```python
from build123d import *

# Parameters (mm, degrees)
BOSS_EXTRUDE1_DEPTH = 4
BOSS_EXTRUDE3_DEPTH = 12


with BuildPart() as part:
    # Sketch1 → Boss-Extrude1 (new body)
    with BuildSketch(Plane(origin=(0, 0, 0), x_dir=(1, 0, 0), z_dir=(0, 1, 0))):
        Polygon((75, 12), (90, 12), (90, 0), (0, 0), (0, 12), (60, 12), (60, 17), (75, 17), align=None)
    extrude(amount=BOSS_EXTRUDE1_DEPTH)

    # Sketch2 → Boss-Extrude3 (add)
    with BuildSketch(Plane.XY):
        with BuildLine():
            Line((1.10505422, 5), (1.175606581, 6.27259339))
            ThreePointArc((1.175606581, 6.27259339), (1.382253241, 6.881354819), (1.916787536, 7.238519216))
            ThreePointArc((1.916787536, 7.238519216), (2.451321831, 6.881354819), (2.657968491, 6.27259339))
            Line((2.657968491, 6.27259339), (2.728520852, 5))
            ThreePointArc((2.728520852, 5), (3.728520852, 4), (4.728520852, 5))
            Line((4.728520852, 5), (4.799073212, 6.27259339))
            ThreePointArc((4.799073212, 6.27259339), (5.005719872, 6.881354819), (5.540254167, 7.238519216))
            ThreePointArc((5.540254167, 7.238519216), (6.074788462, 6.881354819), (6.281435122, 6.27259339))
            Line((6.281435122, 6.27259339), (6.351987483, 5))
            ThreePointArc((6.351987483, 5), (7.351987483, 4), (8.351987483, 5))
            Line((8.351987483, 5), (8.422539844, 6.27259339))
            ThreePointArc((8.422539844, 6.27259339), (8.629186504, 6.881354819), (9.163720799, 7.238519216))
            ThreePointArc((9.163720799, 7.238519216), (9.698255094, 6.881354819), (9.904901754, 6.27259339))
            Line((9.904901754, 6.27259339), (9.975454114, 5))
            ThreePointArc((9.975454114, 5), (10.975454114, 4), (11.975454114, 5))
            Line((11.975454114, 5), (12.046006475, 6.27259339))
            ThreePointArc((12.046006475, 6.27259339), (12.252653135, 6.881354819), (12.78718743, 7.238519216))
            ThreePointArc((12.78718743, 7.238519216), (13.321721725, 6.881354819), (13.528368385, 6.27259339))
            Line((13.528368385, 6.27259339), (13.598920746, 5))
            ThreePointArc((13.598920746, 5), (14.598920746, 4), (15.598920746, 5))
            Line((15.598920746, 5), (15.669473107, 6.27259339))
            ThreePointArc((15.669473107, 6.27259339), (15.876119766, 6.881354819), (16.410654062, 7.238519216))
            ThreePointArc((16.410654062, 7.238519216), (16.945188357, 6.881354819), (17.151835017, 6.27259339))
            Line((17.151835017, 6.27259339), (17.222387377, 5))
            ThreePointArc((17.222387377, 5), (18.222387377, 4), (19.222387377, 5))
            Line((19.222387377, 5), (19.292939738, 6.27259339))
            ThreePointArc((19.292939738, 6.27259339), (19.499586398, 6.881354819), (20.034120693, 7.238519216))
            ThreePointArc((20.034120693, 7.238519216), (20.568654988, 6.881354819), (20.775301648, 6.27259339))
            Line((20.775301648, 6.27259339), (20.845854009, 5))
            ThreePointArc((20.845854009, 5), (21.845854009, 4), (22.845854009, 5))
            Line((22.845854009, 5), (22.91640637, 6.27259339))
            ThreePointArc((22.91640637, 6.27259339), (23.123053029, 6.881354819), (23.657587324, 7.238519216))
            ThreePointArc((23.657587324, 7.238519216), (24.19212162, 6.881354819), (24.398768279, 6.27259339))
            Line((24.398768279, 6.27259339), (24.46932064, 5))
            ThreePointArc((24.46932064, 5), (25.46932064, 4), (26.46932064, 5))
            Line((26.46932064, 5), (26.539873001, 6.27259339))
            ThreePointArc((26.539873001, 6.27259339), (26.746519661, 6.881354819), (27.281053956, 7.238519216))
            ThreePointArc((27.281053956, 7.238519216), (27.815588251, 6.881354819), (28.022234911, 6.27259339))
            Line((28.022234911, 6.27259339), (28.092787272, 5))
            ThreePointArc((28.092787272, 5), (29.092787272, 4), (30.092787272, 5))
            Line((30.092787272, 5), (30.163339632, 6.27259339))
            ThreePointArc((30.163339632, 6.27259339), (30.369986292, 6.881354819), (30.904520587, 7.238519216))
            ThreePointArc((30.904520587, 7.238519216), (31.439054883, 6.881354819), (31.645701542, 6.27259339))
            Line((31.645701542, 6.27259339), (31.716253903, 5))
            ThreePointArc((31.716253903, 5), (32.716253903, 4), (33.716253903, 5))
            Line((33.716253903, 5), (33.786806264, 6.27259339))
            ThreePointArc((33.786806264, 6.27259339), (33.993452924, 6.881354819), (34.527987219, 7.238519216))
            ThreePointArc((34.527987219, 7.238519216), (35.062521514, 6.881354819), (35.269168174, 6.27259339))
            Line((35.269168174, 6.27259339), (35.339720535, 5))
            ThreePointArc((35.339720535, 5), (36.339720535, 4), (37.339720535, 5))
            Line((37.339720535, 5), (37.410272895, 6.27259339))
            ThreePointArc((37.410272895, 6.27259339), (37.616919555, 6.881354819), (38.15145385, 7.238519216))
            ThreePointArc((38.15145385, 7.238519216), (38.685988145, 6.881354819), (38.892634805, 6.27259339))
            Line((38.892634805, 6.27259339), (38.963187166, 5))
            ThreePointArc((38.963187166, 5), (39.963187166, 4), (40.963187166, 5))
            Line((40.963187166, 5), (41.033739527, 6.27259339))
            ThreePointArc((41.033739527, 6.27259339), (41.240386186, 6.881354819), (41.774920482, 7.238519216))
            ThreePointArc((41.774920482, 7.238519216), (42.309454777, 6.881354819), (42.516101437, 6.27259339))
            Line((42.516101437, 6.27259339), (42.586653797, 5))
            ThreePointArc((42.586653797, 5), (43.586653797, 4), (44.586653797, 5))
            Line((44.586653797, 5), (44.657206158, 6.27259339))
            ThreePointArc((44.657206158, 6.27259339), (44.863852818, 6.881354819), (45.398387113, 7.238519216))
            ThreePointArc((45.398387113, 7.238519216), (45.932921408, 6.881354819), (46.139568068, 6.27259339))
            Line((46.139568068, 6.27259339), (46.210120429, 5))
            ThreePointArc((46.210120429, 5), (47.210120429, 4), (48.210120429, 5))
            Line((48.210120429, 5), (48.28067279, 6.27259339))
            ThreePointArc((48.28067279, 6.27259339), (48.487319449, 6.881354819), (49.021853745, 7.238519216))
            ThreePointArc((49.021853745, 7.238519216), (49.55638804, 6.881354819), (49.763034699, 6.27259339))
            Line((49.763034699, 6.27259339), (49.83358706, 5))
            ThreePointArc((49.83358706, 5), (50.83358706, 4), (51.83358706, 5))
            Line((51.83358706, 5), (51.904139421, 6.27259339))
            ThreePointArc((51.904139421, 6.27259339), (52.110786081, 6.881354819), (52.645320376, 7.238519216))
            ThreePointArc((52.645320376, 7.238519216), (53.179854671, 6.881354819), (53.386501331, 6.27259339))
            Line((53.386501331, 6.27259339), (53.457053692, 5))
            ThreePointArc((53.457053692, 5), (54.457053692, 4), (55.457053692, 5))
            Line((55.457053692, 5), (55.527606052, 6.27259339))
            ThreePointArc((55.527606052, 6.27259339), (55.734252712, 6.881354819), (56.268787007, 7.238519216))
            ThreePointArc((56.268787007, 7.238519216), (56.803321303, 6.881354819), (57.009967962, 6.27259339))
            Line((57.009967962, 6.27259339), (57.080520323, 5))
            ThreePointArc((57.080520323, 5), (58.080520323, 4), (59.080520323, 5))
            Line((59.080520323, 5), (59.151072684, 6.27259339))
            ThreePointArc((59.151072684, 6.27259339), (59.357719344, 6.881354819), (59.892253639, 7.238519216))
            ThreePointArc((59.892253639, 7.238519216), (60.426787934, 6.881354819), (60.633434594, 6.27259339))
            Line((60.633434594, 6.27259339), (60.703986955, 5))
            ThreePointArc((60.703986955, 5), (61.703986955, 4), (62.703986955, 5))
            Line((62.703986955, 5), (62.774539315, 6.27259339))
            ThreePointArc((62.774539315, 6.27259339), (62.981185975, 6.881354819), (63.51572027, 7.238519216))
            ThreePointArc((63.51572027, 7.238519216), (64.050254565, 6.881354819), (64.256901225, 6.27259339))
            Line((64.256901225, 6.27259339), (64.327453586, 5))
            ThreePointArc((64.327453586, 5), (65.327453586, 4), (66.327453586, 5))
            Line((66.327453586, 5), (66.398005947, 6.27259339))
            ThreePointArc((66.398005947, 6.27259339), (66.604652607, 6.881354819), (67.139186902, 7.238519216))
            ThreePointArc((67.139186902, 7.238519216), (67.673721197, 6.881354819), (67.880367857, 6.27259339))
            Line((67.880367857, 6.27259339), (67.950920217, 5))
            ThreePointArc((67.950920217, 5), (68.950920217, 4), (69.950920217, 5))
            Line((69.950920217, 5), (70.021472578, 6.27259339))
            ThreePointArc((70.021472578, 6.27259339), (70.228119238, 6.881354819), (70.762653533, 7.238519216))
            ThreePointArc((70.762653533, 7.238519216), (71.297187828, 6.881354819), (71.503834488, 6.27259339))
            Line((71.503834488, 6.27259339), (71.574386849, 5))
            ThreePointArc((71.574386849, 5), (72.574386849, 4), (73.574386849, 5))
            Line((73.574386849, 5), (73.64493921, 6.27259339))
            ThreePointArc((73.64493921, 6.27259339), (73.851585869, 6.881354819), (74.386120165, 7.238519216))
            ThreePointArc((74.386120165, 7.238519216), (74.92065446, 6.881354819), (75.127301119, 6.27259339))
            Line((75.127301119, 6.27259339), (75.19785348, 5))
            ThreePointArc((75.19785348, 5), (76.19785348, 4), (77.19785348, 5))
            Line((77.19785348, 5), (77.268405841, 6.27259339))
            ThreePointArc((77.268405841, 6.27259339), (77.475052501, 6.881354819), (78.009586796, 7.238519216))
            ThreePointArc((78.009586796, 7.238519216), (78.544121091, 6.881354819), (78.750767751, 6.27259339))
            Line((78.750767751, 6.27259339), (78.821320112, 5))
            ThreePointArc((78.821320112, 5), (79.821320112, 4), (80.821320112, 5))
            Line((80.821320112, 5), (80.891872473, 6.27259339))
            ThreePointArc((80.891872473, 6.27259339), (81.098519132, 6.881354819), (81.633053427, 7.238519216))
            ThreePointArc((81.633053427, 7.238519216), (82.167587723, 6.881354819), (82.374234382, 6.27259339))
            Line((82.374234382, 6.27259339), (82.444786743, 5))
            ThreePointArc((82.444786743, 5), (83.444786743, 4), (84.444786743, 5))
            Line((84.444786743, 5), (84.515339104, 6.27259339))
            ThreePointArc((84.515339104, 6.27259339), (84.721985764, 6.881354819), (85.256520059, 7.238519216))
            ThreePointArc((85.256520059, 7.238519216), (85.791054354, 6.881354819), (85.997701014, 6.27259339))
            Line((85.997701014, 6.27259339), (86.068253375, 5))
            ThreePointArc((86.068253375, 5), (86.361146593, 4.292893219), (87.068253375, 4))
            Line((87.068253375, 4), (87.068253375, 1.902319502))
            Line((87.068253375, 1.902319502), (0.10505422, 2.313670855))
            Line((0.10505422, 2.313670855), (0.10505422, 4))
            ThreePointArc((0.10505422, 4), (0.812161001, 4.292893219), (1.10505422, 5))
        make_face()
    extrude(amount=-BOSS_EXTRUDE3_DEPTH)


solid = part.part
```
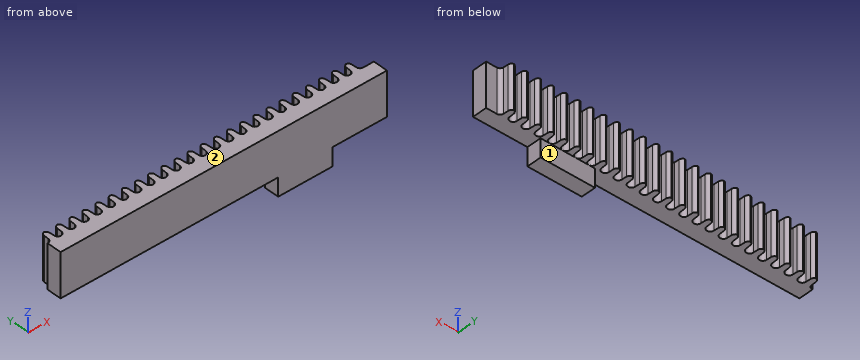
Build history of the part. All positions in model axes, mm. Face numbers are marked on the shaded views. A direction names the side the tool comes from. Give positions to 0.01 mm unless a question says otherwise; leave off trailing zeros. Loops run counter-clockwise (first coordinate to the right, second up) from the corner with the lowest first, then second, coordinate; pieces in that order, holes last.
1) Probe line 1 along Z through (x, y) = (82.5, 4.5); line 2 along X through (y, z) = (3.75, -15); line 3 along Y through (x, z) = (25, -7). List the from-to ranges inside material, lowest first.
Values follow:
line 1: z = -12 to 0
line 2: x = 60 to 75
line 3: y = 0 to 4.12
2) Band-saw the part on A-A on y = 3. List the corners of the cut face in (x, z).
Values follow:
outline: (0, -12) - (60, -12) - (60, -17) - (75, -17) - (75, -12) - (90, -12) - (90, 0) - (0, 0) - close
3) Band-saw the part on B-B on z = -15.25. List the corners of the cut face in (x, y).
Values follow:
outline: (60, 0) - (75, 0) - (75, 4) - (60, 4) - close
4) 3-axis set-ups, long thin cutter, end or side, ignore diameter. For the marked faces 1 and 2: which of +Z, -Z, +X, -X, +Y, -Y reach the whole face in a straight line?
Values follow:
face 1: -Z, +X, -X, +Y
face 2: +Z, +X, -X, +Y, -Y
5) Drop flat-ended pins along their axis: P1, Ø1.6, axis at x = 66.5, y = 6, coming from the -Z side; P2, Ø1.2, axis at y = 1, z = -15.5, coming from the -X side; P3, Ø1.5, axis at x = 67, z = -15.5, coming from the +Y side. Give the stop position or say it passes through.
Values follow:
P1: stops at z = -12
P2: stops at x = 60
P3: stops at y = 4
